Input: dimensioned drawing with shaded views. Units: mm. Origin: part minimum x, y, z. Give positions to 0.01 mm unless a question says otherwise; leave off trailing zeros. Order: outer loops, then holes, each group sorted by start corner. A loop starts at its lowest first (then second) coordinate and runs counter-clockwise, first axis right, second up.
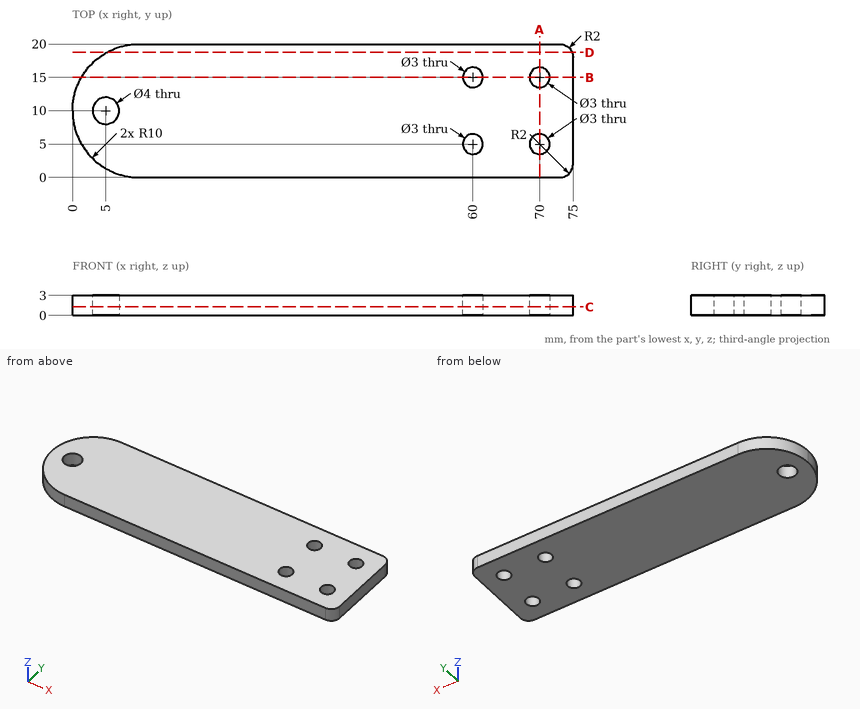
1) Pin query (flat end, axial travel): pin 1 (1.8 mm diameter, centred on x = 70, y = 5, fed in from +Z); pin 2 (2 mm diameter, centred on x = 19.5, y = 8.5, fed in from -Z). Return the tip coordinate at first contact, or that it passes through.
Report:
pin 1: passes through
pin 2: stops at z = 0
2) Section query B-B, the plane y = 15. Return the cut outline in (x, z).
Report:
outline: (1.34, 0) - (58.5, 0) - (58.5, 3) - (1.34, 3) - close; (61.5, 0) - (68.5, 0) - (68.5, 3) - (61.5, 3) - close; (71.5, 0) - (75, 0) - (75, 3) - (71.5, 3) - close
3) Section query C-C, the plane z = 1.3. Count the separate pieces of the cut face and the enclosed holes in it, and give its area (3 significant figures).
Report:
separate pieces: 1
enclosed holes: 5
area: 1,410 mm2
4) Section query D-D, the plane y = 18.75. Return the cut outline in (x, z), and give its area (3 significant figures).
Report:
outline: (5.16, 0) - (74.85, 0) - (74.85, 3) - (5.16, 3) - close
area: 209 mm2
5) Material intervals for L1, parallel to Y at x = 70, z = 1.4; L2, parallel to X at y = 5.5, z = 0.9; L3, parallel to Y at x = 59.5, z = 0.7, sorted ascending.
Report:
L1: y = 0 to 3.5, 6.5 to 13.5, 16.5 to 20
L2: x = 1.07 to 58.59, 61.41 to 68.59, 71.41 to 75
L3: y = 0 to 3.59, 6.41 to 13.59, 16.41 to 20
6) Section query A-A, the plane x = 70. Return the cut outline in (y, z).
Report:
outline: (0, 0) - (3.5, 0) - (3.5, 3) - (0, 3) - close; (6.5, 0) - (13.5, 0) - (13.5, 3) - (6.5, 3) - close; (16.5, 0) - (20, 0) - (20, 3) - (16.5, 3) - close
